Autodesk Inventor part; units mm, degrees
ref_plane "YZ Plane" through (0, 0, 0) normal (1, 0, 0) x (0, 1, 0)
ref_plane "XZ Plane" through (0, 0, 0) normal (0, 1, 0) x (-1, 0, 0)
ref_plane "XY Plane" through (0, 0, 0) normal (0, 0, 1) x (1, 0, 0)
sketch "スケッチ1" plane through (0, 0, 0) normal (0, 1, 0) x (-1, 0, 0)
  line L0 (0, 0) -> (-30, 0)
  line L1 (-30, 0) -> (-30, -250)
  line L2 (-30, -250) -> (0, -250)
  line L3 (0, -250) -> (0, 0)
  point P0 (-15, -12)
  dimension "d0" = 250
  dimension "d1" = 30
  dimension "d4" = 15
  dimension "d5" = 12
extrude "押し出し1" add sketch "スケッチ1" along normal blind 5
sketch "スケッチ2" plane through (0, 0, 0) normal (0, -1, 0) x (1, 0, 0)
  line L0 (0, -250) -> (0, 0)
  line L1 (0, 0) -> (30, 0)
  point P0 (15, -12)
  dimension "d6" = 15
  dimension "d7" = 12
hole "穴1" at (15, 0, -12) direction (0, 1, 0) diameter 11 end through all
sketch "スケッチ3" plane through (0, 0, 0) normal (0, -1, 0) x (1, 0, 0)
  line L0 (0, 0) -> (30, 0)
  circle A0 centre (15, -12) radius 4
  point P0 (23.5, -12)
  point P1 (15, -3.5)
  point P2 (6.5, -12)
  point P3 (15, -20.5)
  dimension "d17" = 360
hole "穴2" at (23.5, 0, -12) at (15, 0, -3.5) at (6.5, 0, -12) at (15, 0, -20.5) direction (0, 1, 0) diameter 3 end through all
sketch "スケッチ4" plane through (0, 0, -250) normal (-1, 0, 0) x (0, 0, 1)
  line L0 (0, 5) -> (250, 5)
  line L1 (0, 0) -> (0, 5)
  point P0 (250, 0)
  point P1 (180, 2.5)
  point P2 (20, 2.5)
  dimension "d25" = 2.5
  dimension "d26" = 180
  dimension "d27" = 20
hole "穴3" at (0, 2.5, -70) at (0, 2.5, -230) direction (1, 0, 0) diameter 2.459 end through all
properties part number "横長3rdフラットバー" material "アルミニウム 6061"
Read the model definition and answer for the solid it produces. Units are mm, in the model's axes. Round coordinates to 2 decimals unless told otherwise and drop trailing zeros. Loops run counter-clockwise (first coordinate to the right, second up) from the corner with the lowest first, then second, coordinate; pieces in that order, holes last. Notation, with made-up numbers: (35.5, -29.75) - (89.5, -29.75) arc R15 ccw to (89.5, -16.75) - close; hole circle Ø5 at (59, 5.5). An arc over 180 degrees is marked (long way). One line per question, with ' | ' between items. Start each with the question number.
Q1. For a pull along X with two mould halves and no side action, classify faces 1 (the cylindrical face through (17.11, 2.54, -17.08)), 2 (the flat face through (15, 2, 0)), 3 (the flat face through (0, 2, -127)) as +X half, -X half, draft (parallel to the pull), parting line (faces both ways), or undercut.
Q2. A flat-ended cylindrical pin translates along its axis: pin 1 (1.5 mm diameter, centred on y = 2.5, z = -230, fed in from +X). Find the tip coordinate at first contact, or state that the pin passes through.
Q3. Find the intervals of material crossed by L1, parallel to X at y = 3.6, z = -12; L2, parallel to Z at x = 23.5, y = 2.2; L3, parallel to Y at x = 27.5, z = -230, in increasing order.
Q4. Section A-A on y = 2.5 is taken. Give the vertices of the cut face in (x, z), plus the area to 3 significant figures.
Established:
1) face 1: undercut | face 2: draft | face 3: -X half
2) pin 1: through
3) L1: 0 to 5, 8 to 9.5, 20.5 to 22, 25 to 30 | L2: -250 to -231.19, -228.81 to -71.19, -68.81 to -13.5, -10.5 to 0 | L3: 0 to 1.27, 3.73 to 5
4) outline: (0, -250) - (30, -250) - (30, -231.23) - (0, -231.23) - close; (0, -228.77) - (30, -228.77) - (30, -71.23) - (0, -71.23) - close; (0, -68.77) - (30, -68.77) - (30, 0) - (0, 0) - close; hole circle Ø3 at (6.5, -12); hole circle Ø11 at (15, -12); hole circle Ø3 at (15, -20.5); hole circle Ø3 at (15, -3.5); hole circle Ø3 at (23.5, -12) | area: 7,230 mm²
